```python
from build123d import *

# Parameters (mm, degrees)
SKETCH1_R           = 100
SKETCH1_R_2         = 1.75
BOSS_EXTRUDE1_DEPTH = 3
BOSS_EXTRUDE2_DEPTH = 2


with BuildPart() as part:
    # Sketch1 → Boss-Extrude1 (new body)
    with BuildSketch(Plane.XY):
        Circle(SKETCH1_R)
        Circle(SKETCH1_R_2, mode=Mode.SUBTRACT)
    extrude(amount=BOSS_EXTRUDE1_DEPTH)

    # Sketch2 → Boss-Extrude2 (add)
    with BuildSketch(Plane.XY.offset(3)):
        Polygon((-3, -77), (-5, -75), (5, -75), (3, -77), align=None)
        Polygon((-58.330554744, -50.354209191), (-63.803375122, -54.718637804), (-63.338227, -56.90579057), (-55.519912176, -50.670892552), align=None)
        Polygon((-91.335858635, 17.769663121), (-84.51136325, 16.212016584), (-83.981477205, 14.039639825), (-93.730756327, 16.264849165), align=None)
        Polygon((-43.054094342, 82.488453498), (-45.723799556, 83.422623755), (-36.714110877, 87.761461146), (-37.648281134, 85.091755932), align=None)
        Polygon((43.054094342, 82.488453498), (45.723799556, 83.422623755), (41.384962165, 74.412935076), (40.016908168, 76.181671422), align=None)
        Polygon((82.561507425, 15.766974716), (83.981477205, 14.039639825), (74.232198083, 11.814430486), (75.73701204, 14.209328178), align=None)
        Polygon((69.573125019, -49.087475746), (69.107976898, -51.274628512), (65.367038087, -55.965617407), (63.338227, -56.90579057), (63.803375122, -54.718637804), (67.544313933, -50.027648909), align=None)
    extrude(amount=BOSS_EXTRUDE2_DEPTH)


solid = part.part
```
The listing builds one solid part. Answer for the finished solid, in the listing's coordinates (mm). A direction names the side the tool comes from. Give positions to 0.01 mm unless a question says otherwise; leave off trailing zeros. Order: outer loops, then holes, each group sorted by start corner. A loop starts at its lowest first (then second) coordinate and runs counter-clockwise, first axis right, second up.
1) Given P1, Ø1, axis at x = -38, z = 4, coming from the +Y side; P2, Ø4, axis at x = 0, y = 0, coming from the +Z side; P3, Ø0.6, axis at x = -2.5, z = 3.5, coming from the +Y side; P4, Ø12, axis at x = -37, y = -67.5, coming from the -Z side, each flat-ended and moving along its own axis, determine where each tip first touches the part or whether it passes through.
Reported:
P1: stops at y = 87.38
P2: stops at z = 3
P3: stops at y = -75
P4: stops at z = 0
2) Find section C-C on y = -40.5. Write down the section's boundary in (x, z).
Reported:
outline: (-91.43, 0) - (91.43, 0) - (91.43, 3) - (-91.43, 3) - close
3) Find section A-A on z = 1.15. Write down the section's boundary in (x, y), then the cut area to 3 significant figures.
Reported:
outline: circle Ø200 at (0, 0); hole circle Ø3.5 at (0, 0)
area: 31,400 mm2
4) For faces 1 (the face through (-41, 85, 5)), 2 (the face through (-41.282, 85.562, 3.986)), determine the directions among +Z, -Z, +X, -X, +Y, -Y from which every point of the face is accessible in a straight line to the end or side of a thin tool.
Reported:
face 1: +Z, +X, -X, +Y, -Y
face 2: +Z, -X, +Y
5) Determine the mould class of faces 3 (the face through (-59.48, -53.83, 3.99)), 4 (the face through (-1.4, 1.4, 0)), 5 (the face through (43.585, 78.981, 3.986)), 6 (the face through (-61.029, -52.506, 3.986)) for opening direction X: pulls with the +X half, pulls with the -X half, needs draft (parallel to the pull), parting line crosses it, or undercut.
Reported:
face 3: undercut
face 4: needs draft
face 5: pulls with the +X half
face 6: pulls with the -X half
6) Consider line 1 along Y through (x, z) = (0, 0.9); line 2 along Z through (x, y) = (-32, 90.5); line 3 along Y through (x, z) = (3, 2.1). Determine where each line is inside the solid, lowest interval first.
Reported:
line 1: y = -100 to -1.75, 1.75 to 100
line 2: z = 0 to 3
line 3: y = -99.95 to 99.95
7) Find section B-B on x = -50. Write down the section's boundary in (y, z).
Reported:
outline: (-86.6, 0) - (86.6, 0) - (86.6, 3) - (-86.6, 3) - close
